```python
from build123d import *

# Parameters (mm, degrees)
BOSS_EXTRUDE1_DEPTH = 5
CUT_EXTRUDE1_DEPTH  = 10


with BuildPart() as part:
    # Sketch1 → Boss-Extrude1 (new body)
    with BuildSketch(Plane.XY):
        Polygon((-12.5, 35), (-12.5, -35), (-2.5, -35), (-2.5, -40), (2.5, -40), (2.5, -35), (12.5, -35), (12.5, 35), (2.5, 35), (2.5, 40), (-2.5, 40), (-2.5, 35), align=None)
    extrude(amount=BOSS_EXTRUDE1_DEPTH)

    # Sketch2 → Cut-Extrude1 (cut)
    with BuildSketch(Plane(origin=(0, 0, 0), x_dir=(-1, 0, 0), z_dir=(0, 0, -1))):
        Polygon((5.8, 35), (9.2, 35), (9.2, 30), (10.25, 30), (10.25, 27.6), (9.2, 27.6), (9.2, 20), (5.8, 20), (5.8, 27.6), (4.75, 27.6), (4.75, 30), (5.8, 30), align=None)
        Polygon((-5.8, 35), (-5.8, 30), (-4.75, 30), (-4.75, 27.6), (-5.8, 27.6), (-5.8, 20), (-9.2, 20), (-9.2, 27.6), (-10.25, 27.6), (-10.25, 30), (-9.2, 30), (-9.2, 35), align=None)
        Polygon((-5.8, -35), (-9.2, -35), (-9.2, -30), (-10.25, -30), (-10.25, -27.6), (-9.2, -27.6), (-9.2, -20), (-5.8, -20), (-5.8, -27.6), (-4.75, -27.6), (-4.75, -30), (-5.8, -30), align=None)
        Polygon((5.8, -35), (5.8, -30), (4.75, -30), (4.75, -27.6), (5.8, -27.6), (5.8, -20), (9.2, -20), (9.2, -27.6), (10.25, -27.6), (10.25, -30), (9.2, -30), (9.2, -35), align=None)
    extrude(amount=-CUT_EXTRUDE1_DEPTH, mode=Mode.SUBTRACT)


solid = part.part
```
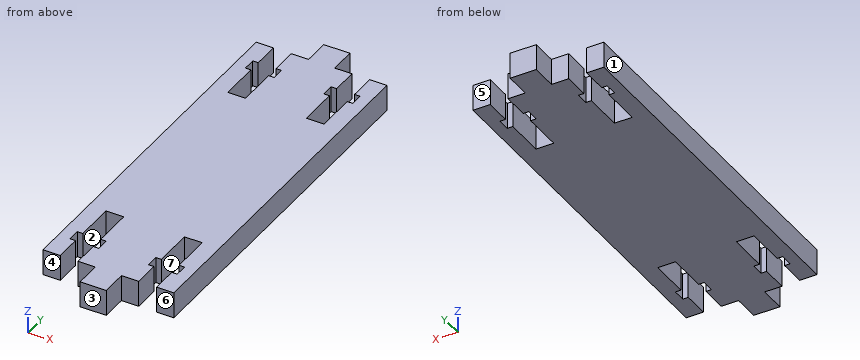
Part model, mm, in its own coordinate system. Face numbers are marked on the shaded views. A direction names the side the tool comes from. Round coordinates to 2 decimals unless told otherwise and drop trailing zeros. Loops run counter-clockwise (first coordinate to the right, second up) from the corner with the lowest first, then second, coordinate; pieces in that order, holes last. Notation, with made-up numbers: (-27, 81.5) -> (-11, 81.5) arc R23 cw to (-11, 103.5) -> close; hole circle Ø10 at (85, -4). An arc over 180 degrees is marked (long way). Use a Markdown table: item, result.
1) Pull direction X, two halves, no side cores. Call the marked faces 1, 2 and 3: pulls with the +X half, pulls with the -X half, needs draft (parallel to the pull), parting line crosses it, or undercut.
The answers:
| item | result |
|---|---|
| face 1 | pulls with the -X half |
| face 2 | undercut |
| face 3 | needs draft |
2) Tool access for the marked faces 4, 5, 6 and 7: list every direction of +Z, -Z, +X, -X, +Y, -Y with a clear straight run to the whole face (end or side of a thin tool).
The answers:
| item | result |
|---|---|
| face 4 | +Z, -Z, -X, -Y |
| face 5 | +Z, -Z, +X, +Y |
| face 6 | +Z, -Z, +X, -Y |
| face 7 | +Z, -Z, -Y |
3) Probe line 1 (Y direction, x = -5, z = 2.05); line 2 (X direction, y = 29.5, z = 0.2); line 3 (Y direction, x = -3, z = 4.75). List the from-to ranges inside material, lowest first. Write a range as [from, to].
The answers:
| item | result |
|---|---|
| line 1 | y = [-35, -30], [-27.6, 27.6], [30, 35] |
| line 2 | x = [-12.5, -10.25], [-4.75, 4.75], [10.25, 12.5] |
| line 3 | y = [-35, 35] |
4) Drop flat-ended pins along their axis: pin 1 Ø2.5 at (x, z) = (-7, 3.5) entering from -Y; pin 2 Ø1 at (x, z) = (-8, 3) entering from +Y; pin 3 Ø2.5 at (x, z) = (-4.5, 3) entering from +Y. Give the stop position or say it passes through.
The answers:
| item | result |
|---|---|
| pin 1 | stops at y = -35 |
| pin 2 | stops at y = 20 |
| pin 3 | stops at y = 35 |
5) Cut at A-A, the plane y = 28.5. List the corners of the cut face in (x, z), and give its area (3 significant figures).
The answers:
| item | result |
|---|---|
| outline | (-12.5, 0) -> (-10.25, 0) -> (-10.25, 5) -> (-12.5, 5) -> close; (-4.75, 0) -> (4.75, 0) -> (4.75, 5) -> (-4.75, 5) -> close; (10.25, 0) -> (12.5, 0) -> (12.5, 5) -> (10.25, 5) -> close |
| area | 70.0 mm2 |
